Part print with two shaded views. Sizes in mm from the minimum x, y, z corner. Round coordinates to 2 decimals unless told otherwise and drop trailing zeros. Loops run counter-clockwise (first coordinate to the right, second up) from the corner with the lowest first, then second, coordinate; pieces in that order, holes last.
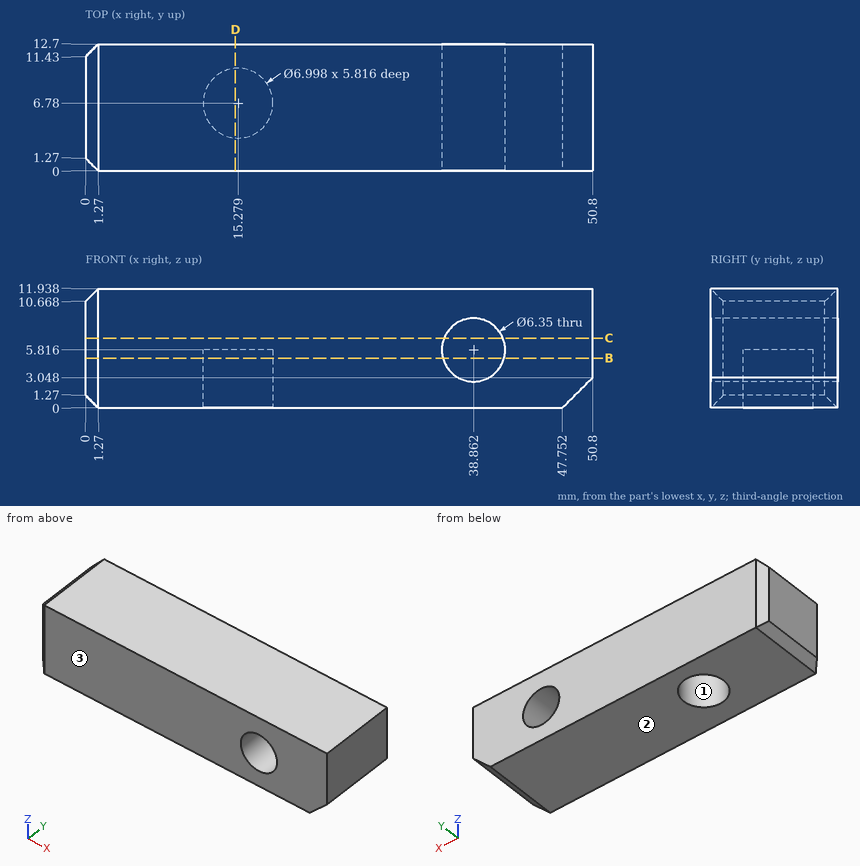
Item 1: Wall check: L1, parallel to X at y = 7.5, z = 6; L2, parallel to Z at x = 18, y = 7.25 (1 decimal); L3, parallel to X at y = 9, z = 5.5 (1 decimal). Give the ranges that are in metal, low to high.
Verdict:
L1: x = 0 to 35.69, 42.03 to 50.8
L2: z = 5.8 to 11.9
L3: x = 0 to 12.6, 18 to 35.7, 42 to 50.8
Item 2: Cut at D-D (x = 15). List the corners of the cut face in (y, z) (1 decimal).
Verdict:
outline: (0, 0) - (3.3, 0) - (3.3, 5.8) - (10.3, 5.8) - (10.3, 0) - (12.7, 0) - (12.7, 11.9) - (0, 11.9) - close
Item 3: Mould opens along Y. For the marked faces 1, 2 and 3 say: released by +Y, released by -Y, zero draft, split by the parting line, or undercut.
Verdict:
face 1: undercut
face 2: zero draft
face 3: released by -Y
Item 4: Cut at C-C (z = 7). List the corners of the cut face in (x, y) (1 decimal).
Verdict:
outline: (0, 1.3) - (1.3, 0) - (35.9, 0) - (35.9, 12.7) - (1.3, 12.7) - (0, 11.4) - close; (41.8, 0) - (50.8, 0) - (50.8, 12.7) - (41.8, 12.7) - close
Item 5: Flat gauge pin, fed straight in: P1, Ø5.5, axis at x = 15.28, y = 6.78, coming from the -Z side. Where does the tip first touch, or does it go through?
Verdict:
P1: stops at z = 5.82
Item 6: Cut at B-B (z = 5). List the corners of the cut face in (x, y), plus the area to 3 significant figures.
Verdict:
outline: (0, 1.27) - (1.27, 0) - (35.79, 0) - (35.79, 12.7) - (1.27, 12.7) - (0, 11.43) - close; (41.93, 0) - (50.8, 0) - (50.8, 12.7) - (41.93, 12.7) - close; hole circle Ø7 at (15.28, 6.78)
area: 527 mm2
